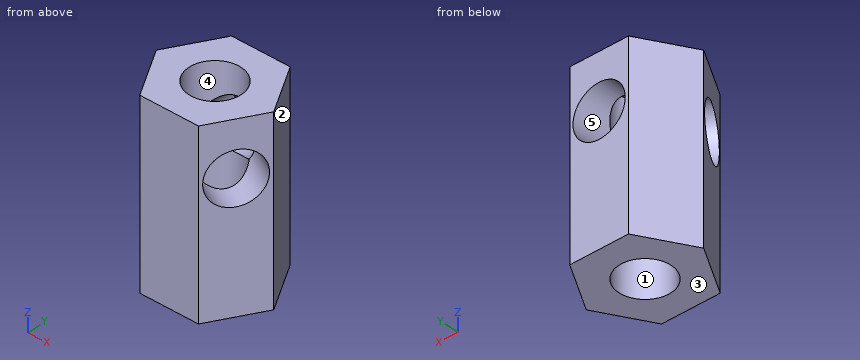
from build123d import *

# Parameters (mm, degrees)
F0_R           = 7.3406
F1_DEPTH       = 25.4
F5_D           = 14.6812
F5_DEPTH       = 16.51
F5_TIP         = 4.41067746
F5_ON_F2_D     = 14.6812
F5_ON_F2_DEPTH = 16.51
F5_ON_F2_TIP   = 4.41067746
F5_ON_F4_D     = 14.6812
F5_ON_F4_DEPTH = 16.51
F5_ON_F4_TIP   = 4.41067746


with BuildPart() as f1:
    # F0 (on Top) → F1 (new body, symmetric)
    with BuildSketch(Plane.XY):
        Polygon((8.248891971, 14.2875), (-8.248891971, 14.2875), (-16.4977839421, 0), (-8.248891971, -14.2875), (8.248891971, -14.2875), (16.4977839421, 0), align=None)
        Circle(F0_R, mode=Mode.SUBTRACT)
    extrude(amount=F1_DEPTH, both=True)

    # F5
    with Locations(Plane(origin=(0, 14.2875, 0), x_dir=(-1, 0, 0), z_dir=(0, 1, 0))):
        with Locations((0, 10.16)):
            Hole(F5_D / 2, depth=F5_DEPTH)
            with Locations((0, 0, -(F5_DEPTH + F5_TIP / 2))):  # 118° drill point
                Cone(0, F5_D / 2, F5_TIP, mode=Mode.SUBTRACT)

    # F5 on F2
    with Locations(Plane(origin=(12.3733379566, -7.14375, 0), x_dir=(0.5, 0.8660254038, 0), z_dir=(0.8660254038, -0.5, 0))):
        with Locations((0, 10.16)):
            Hole(F5_ON_F2_D / 2, depth=F5_ON_F2_DEPTH)
            with Locations((0, 0, -(F5_ON_F2_DEPTH + F5_ON_F2_TIP / 2))):  # 118° drill point
                Cone(0, F5_ON_F2_D / 2, F5_ON_F2_TIP, mode=Mode.SUBTRACT)

    # F5 on F4
    with Locations(Plane(origin=(-12.3733379566, -7.14375, 0), x_dir=(0.5, -0.8660254038, 0), z_dir=(-0.8660254038, -0.5, 0))):
        with Locations((0, 10.16)):
            Hole(F5_ON_F4_D / 2, depth=F5_ON_F4_DEPTH)
            with Locations((0, 0, -(F5_ON_F4_DEPTH + F5_ON_F4_TIP / 2))):  # 118° drill point
                Cone(0, F5_ON_F4_D / 2, F5_ON_F4_TIP, mode=Mode.SUBTRACT)


solid = f1.part
Design review of the part built by this model. Coordinates are the model's own, in mm. Face numbers are marked on the shaded views. A direction names the side the tool comes from. Give positions to 0.01 mm unless a question says otherwise; leave off trailing zeros. Order: outer loops, then holes, each group sorted by start corner. A loop starts at its lowest first (then second) coordinate and runs counter-clockwise, first axis right, second up. Notation, with made-up numbers: (50.25, 56) - (66.25, 56) arc R20 cw to (66.25, 74) - close; hole circle Ø3 at (-17, -2.5). An arc over 180 degrees is marked (long way). Write item = value, one per line. Start each with the question number.
Q1. We need section A-A on z = 0. State the section outline as (x, y) points.
Q2. We need section C-C on y = 10.25. State the section outline as (x, z) points, plus the area to 3 significant figures.
Q3. To check wall thickness, follow L1, parallel to Y at x = 0, z = -9; L2, parallel to Z at x = 0, y = 12.25; L3, parallel to X at y = 0, z = 19.25. State the ranges of each line that lie inside material, in increasing order. Write a range as from..to.
Q4. Clearance check with flat-ended pins moving along their axes: pin 1 Ø5 at (y, z) = (-8.5, 10) entering from +X; pin 2 Ø3 at (y, z) = (10.5, -9) entering from +X; pin 3 Ø1.5 at (y, z) = (-6.5, -3.5) entering from -X. State where each tip first meets the part, or that it passes through.
Q5. Tool access review of the marked faces 4 and 5: name each direction out of +Z, -Z, +X, -X, +Y, -Y from which nothing blocks a thin tool from reaching the whole face with its end or side.
Q6. Mouldability with a two-part tool opening along X and no side actions: class the marked faces 1, 2 and 3 as released by +X, released by -X, zero draft, split by the parting line, or undercut.
Q7. We need section D-D on x = -2.5. State how many separate pieces and enclosed holes the cut face has, plus the area to 3 significant figures.
Q8. We need section B-B on z = 10.16. State the section outline as (x, y) points.
Working result:
q1.outline = (-16.5, 0) - (-8.25, -14.29) - (8.25, -14.29) - (16.5, 0) - (8.25, 14.29) - (-8.25, 14.29) - close; hole circle Ø14.68 at (0, 0)
q2.outline = (-10.58, -25.4) - (10.58, -25.4) - (10.58, 25.4) - (-10.58, 25.4) - close; hole circle Ø14.68 at (0, 10.16)
q2.area = 906 mm²
q3.L1 = -14.29..-7.34, 7.34..14.29
q3.L2 = -25.4..2.82, 17.5..25.4
q3.L3 = -16.5..-7.34, 7.34..16.5
q4.pin_1 = 4.38
q4.pin_2 = 11.3
q4.pin_3 = -13.18
q5.face_4 = +Z, -Z
q5.face_5 = +Y
q6.face_1 = undercut
q6.face_2 = released by +X
q6.face_3 = zero draft
q7.separate_pieces = 3
q7.enclosed_holes = 0
q7.area = 625 mm²
q8.outline = (-16.5, 0) - (-16.04, -0.79) - (-7.34, 4.24) - (-7.34, 14.29) - (-8.25, 14.29) - close; (-8.7, -13.5) - (-8.25, -14.29) - (8.25, -14.29) - (8.7, -13.5) - (0, -8.48) - close; (7.34, 4.24) - (16.04, -0.79) - (16.5, 0) - (8.25, 14.29) - (7.34, 14.29) - close
